CAD build for the part. Positions are in the model's coordinates, mm. Face numbers are marked on the shaded views. A direction names the side the tool comes from. Round coordinates to 2 decimals unless told otherwise and drop trailing zeros. Order: outer loops, then holes, each group sorted by start corner. A loop starts at its lowest first (then second) coordinate and runs counter-clockwise, first axis right, second up. Notation, with made-up numbers: M 69,15.25 L 106,15.25 A12 cw 106,37.25 Z; hole C 57.25,30.25 d3. An arc over 180 degrees is marked long. Answer as CSV lines item,"result". Start each with the question number.
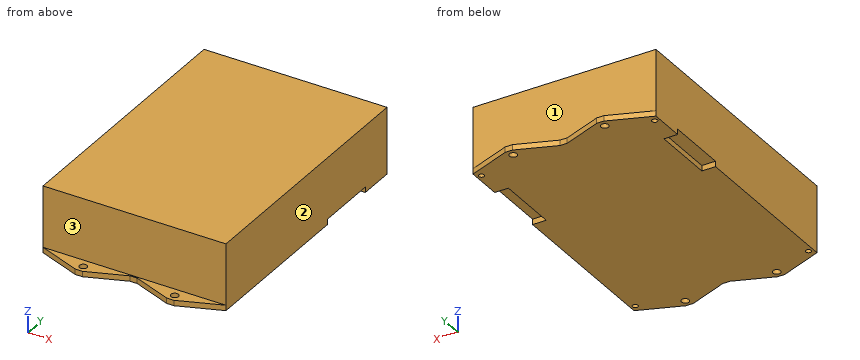
```python
from build123d import *

# Parameters (mm, degrees)
ESQUISSE1_R        = 2.1
ESQUISSE1_R_2      = 1.5
BOSS_EXTRU_1_DEPTH = 3
ESQUISSE2_W        = 101.6
ESQUISSE2_H        = 146.3
BOSS_EXTRU_2_DEPTH = 34


with BuildPart() as part:
    # Esquisse1 → Boss.-Extru.1 (new body)
    with BuildSketch(Plane.XY):
        Polygon((-50.8, 73.15), (-27.4, 82.15), (-23.4, 82.15), (-2, 73.919230769), (2, 73.919230769), (23.4, 82.15), (27.4, 82.15), (50.8, 73.15), (50.8, 53.45), (43.2, 53.45), (43.2, 19.05), (50.8, 19.05), (50.8, -73.15), (27.4, -82.15), (23.4, -82.15), (2, -73.919230769), (-2, -73.919230769), (-23.4, -82.15), (-27.4, -82.15), (-50.8, -73.15), (-50.8, 19.05), (-43.2, 19.05), (-43.2, 53.45), (-50.8, 53.45), align=None)
        with Locations((-25.4, -78.15)):
            Circle(ESQUISSE1_R, mode=Mode.SUBTRACT)
        with Locations(Location((25.4, -78.15, 0), (0, 0, 180))):
            Circle(ESQUISSE1_R, mode=Mode.SUBTRACT)
        with Locations(Location((-25.4, 78.15, 0), (0, 0, 180))):
            Circle(ESQUISSE1_R, mode=Mode.SUBTRACT)
        with Locations((25.4, 78.15)):
            Circle(ESQUISSE1_R, mode=Mode.SUBTRACT)
        with Locations((-48.1, -69.85)):
            Circle(ESQUISSE1_R_2, mode=Mode.SUBTRACT)
        with Locations(Location((48.1, -69.85, 0), (0, 0, 180))):
            Circle(ESQUISSE1_R_2, mode=Mode.SUBTRACT)
        with Locations(Location((-48.1, 69.85, 0), (0, 0, 180))):
            Circle(ESQUISSE1_R_2, mode=Mode.SUBTRACT)
        with Locations((48.1, 69.85)):
            Circle(ESQUISSE1_R_2, mode=Mode.SUBTRACT)
    extrude(amount=BOSS_EXTRU_1_DEPTH)

    # Esquisse2 → Boss.-Extru.2 (add)
    with BuildSketch(Plane.XY.offset(3)):
        Rectangle(ESQUISSE2_W, ESQUISSE2_H)
    extrude(amount=BOSS_EXTRU_2_DEPTH)


solid = part.part
```
Q1. Probe line 1 along X through (y, z) = (-69.85, 1.25); line 2 along Y through (x, z) = (-25.4, 2.05); line 3 along Y through (x, z) = (48, 2). List the from-to ranges inside material, lowest first. Write a range as from..to.
Q2. Band-saw the part on C-C, the plane x = -9.5. Write the cut outline in (y, z).
Q3. Drop flat-ended pins along their axis: P1, Ø5, axis at x = 25.4, y = -78.15, coming from the +Z side; P2, Ø4, axis at x = -14, y = 59.5, coming from the -Z side; P3, Ø2.5, axis at x = -25.4, y = -78.15, coming from the -Z side; P4, Ø1.5, axis at x = -47, z = 2, coming from the +Y side. Give the stop position or say it passes through.
Q4. Band-saw the part on D-D, the plane z = 14. Write the cut outline in (x, y).
Q5. Band-saw the part on A-A, the plane y = 78.15. Write the cut outline in (x, z), then the cut area to 3 significant figures.
Q6. Tool access for the marked faces 1, 2 and 3: list every direction of +Z, -Z, +X, -X, +Y, -Y with a clear straight run to the whole face (end or side of a thin tool).
Q7. Band-saw the part on B-B, the plane x = -25.4. Write the cut outline in (y, z), then the cut area to 3 significant figures.
Answer:
1,line 1,"x = -50.8..-49.6, -46.6..46.6, 49.6..50.8"
1,line 2,"y = -82.15..-80.25, -76.05..76.05, 80.25..82.15"
1,line 3,"y = -74.23..-71.35, -68.35..19.05, 53.45..68.35, 71.35..74.23"
2,outline,"M -76.8,0 L 76.8,0 L 76.8,3 L 73.15,3 L 73.15,37 L -73.15,37 L -73.15,3 L -76.8,3 Z"
3,P1,"stops at z = 3"
3,P2,"stops at z = 0"
3,P3,"passes through"
3,P4,"stops at y = 74.9"
4,outline,"M -50.8,-73.15 L 50.8,-73.15 L 50.8,73.15 L -50.8,73.15 Z"
5,outline,"M -37.8,0 L -27.5,0 L -27.5,3 L -37.8,3 Z; M -23.3,0 L -13,0 L -13,3 L -23.3,3 Z; M 13,0 L 23.3,0 L 23.3,3 L 13,3 Z; M 27.5,0 L 37.8,0 L 37.8,3 L 27.5,3 Z"
5,area,"124 mm^2"
6,face 1,"+Z, +X, -X, +Y"
6,face 2,"+Z, -Z, +X, +Y, -Y"
6,face 3,"+Z, +X, -X, -Y"
7,outline,"M -82.15,0 L -80.25,0 L -80.25,3 L -82.15,3 Z; M -76.05,0 L 76.05,0 L 76.05,3 L 73.15,3 L 73.15,37 L -73.15,37 L -73.15,3 L -76.05,3 Z; M 80.25,0 L 82.15,0 L 82.15,3 L 80.25,3 Z"
7,area,"5,440 mm^2"
